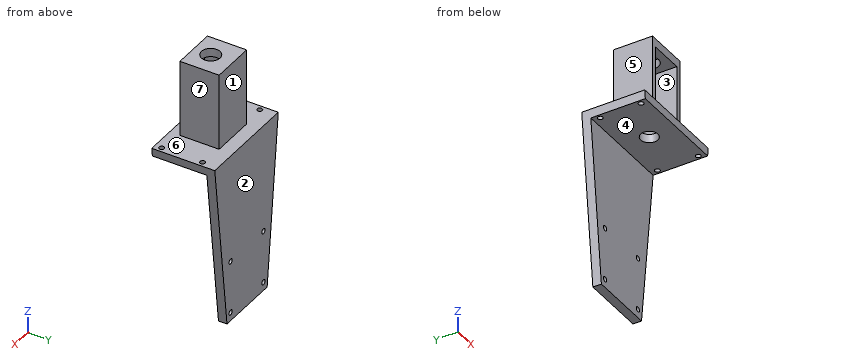
```python
from build123d import *

# Parameters (mm, degrees)
SKETCH1_W           = 60
SKETCH1_H           = 32
BOSS_EXTRUDE1_DEPTH = 5
SKETCH2_R           = 1.5
CUT_EXTRUDE1_DEPTH  = 5
SKETCH4_R           = 5
CUT_EXTRUDE2_DEPTH  = 5
SKETCH5_W           = 60
SKETCH5_H           = 5
BOSS_EXTRUDE2_DEPTH = 100
SKETCH6_R           = 1.5
CUT_EXTRUDE3_DEPTH  = 100
CUT_EXTRUDE4_DEPTH  = 100
BOSS_EXTRUDE3_DEPTH = 45
SKETCH9_W           = 26
SKETCH9_H           = 23
BOSS_EXTRUDE4_DEPTH = 5
SKETCH10_R          = 5.5
CUT_EXTRUDE5_DEPTH  = 5


with BuildPart() as part:
    # Sketch1 → Boss-Extrude1 (new body)
    with BuildSketch(Plane.XY):
        Rectangle(SKETCH1_W, SKETCH1_H)
    extrude(amount=BOSS_EXTRUDE1_DEPTH)

    # Sketch2 → Cut-Extrude1 (cut)
    with BuildSketch(Plane.XY.offset(5)):
        with Locations((27, 12)):
            Circle(SKETCH2_R)
        with Locations((27, -12)):
            Circle(SKETCH2_R)
        with Locations((-27, -12)):
            Circle(SKETCH2_R)
        with Locations((-27, 12)):
            Circle(SKETCH2_R)
    extrude(amount=-CUT_EXTRUDE1_DEPTH, mode=Mode.SUBTRACT)

    # Sketch4 → Cut-Extrude2 (cut)
    with BuildSketch(Plane.XY.offset(5)):
        Circle(SKETCH4_R)
    extrude(amount=-CUT_EXTRUDE2_DEPTH, mode=Mode.SUBTRACT)

    # Sketch5 → Boss-Extrude2 (add)
    with BuildSketch(Plane.XY.offset(5)):
        with Locations((0, 18.5)):
            Rectangle(SKETCH5_W, SKETCH5_H)
    extrude(amount=-BOSS_EXTRUDE2_DEPTH)

    # Sketch6 → Cut-Extrude3 (cut)
    with BuildSketch(Plane.XZ.offset(-16)):
        with Locations(Location((15, -59, 0), (0, 0, 270))):
            Circle(SKETCH6_R)
        with Locations(Location((-16, -59, 0), (0, 0, 270))):
            Circle(SKETCH6_R)
        with Locations(Location((15, -90, 0), (0, 0, 270))):
            Circle(SKETCH6_R)
        with Locations(Location((-16, -90, 0), (0, 0, 270))):
            Circle(SKETCH6_R)
    extrude(amount=-CUT_EXTRUDE3_DEPTH, mode=Mode.SUBTRACT)

    # Sketch7 → Cut-Extrude4 (cut)
    with BuildSketch(Plane(origin=(0, 21, 0), x_dir=(1, 0, 0), z_dir=(0, 1, 0))):
        Polygon((30, -5), (18.449048919, 95), (30, 95), align=None)
        Polygon((-30, -5), (-19.496844987, 95), (-30, 95), align=None)
    extrude(amount=-CUT_EXTRUDE4_DEPTH, mode=Mode.SUBTRACT)

    # Sketch8 → Boss-Extrude3 (add)
    with BuildSketch(Plane.XY.offset(5)):
        Polygon((13, 13), (-13, 13), (-13, -10), (-10, -10), (-10, 10), (10, 10), (10, -10), (13, -10), align=None)
    extrude(amount=BOSS_EXTRUDE3_DEPTH)

    # Sketch9 → Boss-Extrude4 (add)
    with BuildSketch(Plane.XY.offset(50)):
        with Locations((0, 1.5)):
            Rectangle(SKETCH9_W, SKETCH9_H)
    extrude(amount=-BOSS_EXTRUDE4_DEPTH)

    # Sketch10 → Cut-Extrude5 (cut)
    with BuildSketch(Plane.XY.offset(50)):
        Circle(SKETCH10_R)
    extrude(amount=-CUT_EXTRUDE5_DEPTH, mode=Mode.SUBTRACT)


solid = part.part
```
Can you work these out from the model? Positions are in its coordinate system, mm. Face numbers are marked on the shaded views. A direction names the side the tool comes from. Give positions to 0.01 mm unless a question says otherwise; leave off trailing zeros. Order: outer loops, then holes, each group sorted by start corner. A loop starts at its lowest first (then second) coordinate and runs counter-clockwise, first axis right, second up. Notation, with made-up numbers: M -34,-39 L -14,-39 A20 cw -14,-6 Z; hole C 87,33.25 d2. An arc over 180 degrees is marked long. One line per item, written item: value.
1) I want a section at C-C, the plane y = 0. List the corners of the cut face in (x, z) for me, plus the area to 3 significant figures.
Answer sheet:
outline: M -30,5 L -29.47,0 L -5,0 L -5,5 L -10,5 L -10,45 L -5.5,45 L -5.5,50 L -13,50 L -13,5 Z; M 5,0 L 29.42,0 L 30,5 L 13,5 L 13,50 L 5.5,50 L 5.5,45 L 10,45 L 10,5 L 5,5 Z
area: 562 mm^2
2) We'd pull the mould along X, two halves only. Please class the marked faces 5, 6 and 7: released by +X, released by -X, zero draft, split by the parting line, or undercut.
Answer sheet:
face 5: released by -X
face 6: undercut
face 7: released by +X
3) On a 3-axis mill with a long thin cutter (end or side, diameter ignored), from which of +Z, -Z, +X, -X, +Y, -Y can I reach the whole of each face in a straight line? I mean the marked faces 1, 2, 3 and 4. Say none if no direction works.
Answer sheet:
face 1: +Z, +X, -X, +Y
face 2: +Z, -Z, +X, -X, +Y
face 3: -Y
face 4: -Z, +X, -X, -Y
4) Please list where these lines run through material, in increasing order: line 1 along X through (y, z) = (-5.5, 28); line 2 along Y through (x, z) = (-27, 1); line 3 along Z through (x, y) = (-9.5, -2).
Answer sheet:
line 1: x = -13 to -10, 10 to 13
line 2: y = -16 to -13.5, -10.5 to 10.5, 13.5 to 21
line 3: z = 0 to 5, 45 to 50
5) For P1, Ø6, axis at x = 1, y = 1, coming from the -Z side; P2, Ø8, axis at y = 17, z = -74.5, coming from the +X side; P3, Ø16, axis at y = 5, z = 29, coming from the +X side; P4, Ø5, axis at x = -17.5, y = -0.5, coming from the +Z side, each with a flat end and sliding along its axis, tell me the tip position at first contact or that it passes through.
Answer sheet:
P1: passes through
P2: stops at x = 21.28
P3: stops at x = 13
P4: stops at z = 5
6) I want a section at A-A, the plane x = -16. List the corners of the cut face in (y, z) for me.
Answer sheet:
outline: M -16,0 L 16,0 L 16,-57.5 L 21,-57.5 L 21,5 L -16,5 Z; M 16,-95 L 21,-95 L 21,-91.5 L 16,-91.5 Z; M 16,-88.5 L 21,-88.5 L 21,-60.5 L 16,-60.5 Z
7) I want a section at D-D, the plane x = 7. List the corners of the cut face in (y, z) for me.
Answer sheet:
outline: M -16,0 L 16,0 L 16,-95 L 21,-95 L 21,5 L 13,5 L 13,50 L -10,50 L -10,45 L 10,45 L 10,5 L -16,5 Z
8) I want a section at B-B, the plane y = -7. List the corners of the cut face in (x, z) for me, plus the area to 3 significant figures.
Answer sheet:
outline: M -30,5 L -29.47,0 L 29.42,0 L 30,5 L 13,5 L 13,50 L -13,50 L -13,5 Z; hole M -10,5 L 10,5 L 10,45 L -10,45 Z
area: 667 mm^2
